The listing builds one solid part. Answer for the finished solid, in the listing's coordinates (mm). A direction names the side the tool comes from. Round coordinates to 2 decimals unless told otherwise and drop trailing zeros. Order: outer loops, then holes, each group sorted by start corner. A loop starts at its lowest first (then second) coordinate and runs counter-clockwise, first axis right, second up. Notation, with made-up numbers: (67, 0.5) - (80, 0.5) arc R24 cw to (80, 37.5) - close; hole circle Ø3 at (70, 18.5). An arc over 180 degrees is marked (long way). Use CSV: the item, a comma, the result in double quotes. Start each with the question number.
Item 1: Find section C-C, the plane z = 6.35. Count the separate pieces of the cut face and the enclosed holes in it, plus the area to 3 significant figures.
Item 2: Find section B-B, the plane x = -114.3. Give the vertices of the cut face in (y, z) (3 decimals), plus the area to 3 significant figures.
Item 3: Find section A-A, the plane x = -25.4. Give the vertices of the cut face in (y, z) (3 decimals), plus the area to 3 significant figures.
Item 4: Straight lines are drawn through the part: line 1 along Z through (x, y) = (-114, -70); line 2 along X through (y, z) = (-3.5, 12.25); line 3 along Y through (x, z) = (0, 5). For each, find the intervals that lie inside material, in ascending order. Write a range as [from, to].
Item 5: Determine the mould class of faces 5 (the flat face through (-114, -63.5, 6)), 6 (the flat face through (-116, 76.2, 3)), 7 (the flat face through (-2, -21, 12.7)) for opening direction Z: +Z half, -Z half, draft (parallel to the pull), parting line (faces both ways), or undercut.
Item 6: For faces 1 (the flat face through (114, -76.2, 6)), 2 (the flat face through (-114, 63.5, 6)), 3 (the flat face through (101.6, 89, 6)), 4 (the cylindrical face through (109.399, -4.822, 6.261)), determine the directions among +Z, -Z, +X, -X, +Y, -Y from which every point of the face is accessible in a straight line to the end or side of a thin tool.
Item 7: Flat-ended cylindrical pins translate along their axes: P1, Ø6.5, axis at y = -92.5, z = 7.5, coming from the +X side; P2, Ø6.5, axis at y = 90.5, z = 5, coming from the -X side; P3, Ø6, axis at x = -65, y = -7, coming from the -Z side; P4, Ø5, axis at x = -113.5, z = 7.5, coming from the +Y side. Find the tip coordinate at first contact, or state that the pin passes through.
```python
from build123d import *

# Parameters (mm, degrees)
F0_W      = 254
F0_H      = 152.4
F1_DEPTH  = 12.7
F2_W      = 203.2
F2_H      = 12.7
F3_DEPTH  = 25.4
F4_W      = 203.2
F4_H      = 12.7
F5_DEPTH  = 25.4
F6_R      = 3.175
F7_DEPTH  = 12.7
F8_R      = 3.175
F9_DEPTH  = 12.7
F10_W     = 19.05
F10_H     = 12.7
F11_DEPTH = 25.4
F12_R     = 5.08
F13_R     = 3.937
F14_DEPTH = 25.4
F15_R     = 7.9375
F16_DEPTH = 25.4
F17_R     = 3.9624
F18_DEPTH = 25.4
F19_R     = 3.175
F20_DEPTH = 25.4


with BuildPart() as f1:
    # F0 (on Top) → F1 (new body)
    with BuildSketch(Plane.XY):
        Rectangle(F0_W, F0_H)
    extrude(amount=F1_DEPTH)

    # F2 (on face) → F3 (join)
    with BuildSketch(Plane(origin=(0, 76.2, 0), x_dir=(-1, 0, 0), z_dir=(0, 1, 0))):
        with Locations((0, 6.35)):
            Rectangle(F2_W, F2_H)
    extrude(amount=F3_DEPTH)

    # F4 (on face) → F5 (join)
    with BuildSketch(Plane.XZ.offset(76.2)):
        with Locations((0, 6.35)):
            Rectangle(F4_W, F4_H)
    extrude(amount=F5_DEPTH)

    # F6 (on face) → F7 (cut)
    with BuildSketch(Plane.XZ.offset(76.2)):
        with Locations((-114.3, 6.35)):
            Circle(F6_R)
    extrude(amount=-F7_DEPTH, mode=Mode.SUBTRACT)

    # F8 (on face) → F9 (cut)
    with BuildSketch(Plane(origin=(0, 76.2, 0), x_dir=(-1, 0, 0), z_dir=(0, 1, 0))):
        with Locations((114.3, 6.35)):
            Circle(F8_R)
    extrude(amount=-F9_DEPTH, mode=Mode.SUBTRACT)

    # F10 (on face) → F11 (cut)
    with BuildSketch(Plane.XY.offset(12.7)):
        with Locations((117.475, 0)):
            Rectangle(F10_W, F10_H)
    extrude(amount=-F11_DEPTH, mode=Mode.SUBTRACT)

    # F12
    f12_edges = [f1.edges().sort_by_distance(p)[0] for p in [
        (101.6, -101.6, 6.35),
        (127, -76.2, 6.35),
        (127, -6.35, 6.35),
        (127, 6.35, 6.35),
        (107.95, 6.35, 6.35),
        (107.95, -6.35, 6.35),
        (127, 76.2, 6.35),
        (101.6, 76.2, 6.35),
        (101.6, 101.6, 6.35),
        (101.6, -76.2, 6.35),
        (-101.6, -101.6, 6.35),
        (-101.6, -76.2, 6.35),
        (-127, -76.2, 6.35),
        (-127, 76.2, 6.35),
        (-101.6, 76.2, 6.35),
        (-101.6, 101.6, 6.35),
    ]]
    fillet(f12_edges, radius=F12_R)

    # F13 (on face) → F14 (cut)
    with BuildSketch(Plane.XY.offset(12.7)):
        Circle(F13_R)
    extrude(amount=-F14_DEPTH, mode=Mode.SUBTRACT)

    # F15 (on face) → F16 (cut)
    with BuildSketch(Plane.XY.offset(12.7)):
        with Locations((31.9151, 0)):
            Circle(F15_R)
    extrude(amount=-F16_DEPTH, mode=Mode.SUBTRACT)

    # F17 (on face) → F18 (cut)
    with BuildSketch(Plane.XY.offset(12.7)):
        with Locations((-64.36106, 0)):
            Circle(F17_R)
    extrude(amount=-F18_DEPTH, mode=Mode.SUBTRACT)

    # F19 (on face) → F20 (cut)
    with BuildSketch(Plane.XY.offset(12.7)):
        with Locations((-25.4, 0)):
            Circle(F19_R)
    extrude(amount=-F20_DEPTH, mode=Mode.SUBTRACT)


solid = f1.part
```
Worked out:
1,separate pieces,"1"
1,enclosed holes,"4"
1,area,"48,300 mm²"
2,outline,"(-76.2, 0) - (76.2, 0) - (76.2, 3.175) - (63.5, 3.175) - (63.5, 9.525) - (76.2, 9.525) - (76.2, 12.7) - (-76.2, 12.7) - (-76.2, 9.525) - (-63.5, 9.525) - (-63.5, 3.175) - (-76.2, 3.175) - close"
2,area,"1,770 mm²"
3,outline,"(-101.6, 0) - (-3.175, 0) - (-3.175, 12.7) - (-101.6, 12.7) - close; (3.175, 0) - (101.6, 0) - (101.6, 12.7) - (3.175, 12.7) - close"
3,area,"2,500 mm²"
4,line 1,"z = [0, 3.19], [9.51, 12.7]"
4,line 2,"x = [-127, -66.22], [-62.5, -1.8], [1.8, 24.79], [39.04, 108.47]"
4,line 3,"y = [-101.6, -3.94], [3.94, 101.6]"
5,face 5,"undercut"
5,face 6,"draft"
5,face 7,"+Z half"
6,face 1,"+Z, -Z, +X, -Y"
6,face 2,"+Y"
6,face 3,"+Z, -Z, +X, +Y"
6,face 4,"+Z, -Z, +X"
7,P1,"stops at x = 101.6"
7,P2,"stops at x = -101.6"
7,P3,"stops at z = 0"
7,P4,"stops at y = 76.2"
